The listing builds one solid part. Answer for the finished solid, in the listing's coordinates (mm). Face numbers are marked on the shaded views. Round coordinates to 2 decimals unless told otherwise and drop trailing zeros. Loops run counter-clockwise (first coordinate to the right, second up) from the corner with the lowest first, then second, coordinate; pieces in that order, holes last. Notation, with made-up numbers: (60.25, -27.75) -> (108.25, -27.75) arc R25 cw to (108.25, -2.75) -> close; hole circle Ø7 at (34.25, -13). An arc over 180 degrees is marked (long way). Write each question's results on one line, items separated by ' | '. Start each with the question number.
(1) The part is cut by section D-D (z = -4). Determine the outline of the cut face in (x, y), plus the area to 3 significant figures.
(2) Straight lines are drawn through the part: probe 1 along X at (y, z) = (1.8, 39.5); probe 2 along X at (y, z) = (0.7, 42.5); probe 3 along Y at (x, z) = (-6, -43). For each, find the intervals that lie inside material, in ascending order.
(3) The part is cut by section B-B (x = 23.5). Determine the outline of the cut face in (y, z), plus the area to 3 significant figures.
(4) The part is cut by section C-C (y = 3.3). Determine the outline of the cut face in (x, z), plus the area to 3 significant figures.
(5) Flat-ended cylindrical pins translate along their axes: pin 1 (3 mm diameter, centred on x = 13.5, z = -7.5, fed in from +Y); pin 2 (1.8 mm diameter, centred on x = 13.5, z = 42.5, fed in from -Y). Find the tip coordinate at first contact, or state that the pin passes through.
(6) Determine the mould class of the marked faces 1 and 2 for opening direction X: released by +X, released by -X, zero draft, split by the parting line, or undercut.
(7) The part is cut by section A-A (z = 42.5). Determine the outline of the cut face in (x, y).
```python
from build123d import *

# Parameters (mm, degrees)
ESQUISSE1_W             = 66
ESQUISSE1_H             = 104
BOSS_EXTRU_1_DEPTH      = 1.5875
ESQUISSE2_W             = 104
ESQUISSE2_H             = 4
BOSS_EXTRU_2_DEPTH      = 1.5875
ESQUISSE3_W             = 104
ESQUISSE3_H             = 4
BOSS_EXTRU_3_DEPTH      = 1.5875
CONG_2_R                = 2
CONG_3_R                = 2
ESQUISSE4_R             = 1
ENL_V_MAT_EXTRU_1_DEPTH = 1.5875


with BuildPart() as part:
    # Esquisse1 → Boss.-Extru.1 (new body)
    with BuildSketch(Plane(origin=(0, 0, 0), x_dir=(1, 0, 0), z_dir=(0, 1, 0))):
        Rectangle(ESQUISSE1_W, ESQUISSE1_H)
    extrude(amount=BOSS_EXTRU_1_DEPTH)

    # Esquisse2 → Boss.-Extru.2 (add)
    with BuildSketch(Plane.ZY.offset(33)):
        with Locations((0, 2)):
            Rectangle(ESQUISSE2_W, ESQUISSE2_H)
    extrude(amount=BOSS_EXTRU_2_DEPTH)

    # Esquisse3 → Boss.-Extru.3 (add)
    with BuildSketch(Plane(origin=(33, 0, 0), x_dir=(0, 0, -1), z_dir=(1, 0, 0))):
        with Locations((0, 2)):
            Rectangle(ESQUISSE3_W, ESQUISSE3_H)
    extrude(amount=BOSS_EXTRU_3_DEPTH)

    # Congé2
    cong_2_edges = [part.edges().sort_by_distance(p)[0] for p in [
        (34.5875, 0, 0),
    ]]
    fillet(cong_2_edges, radius=CONG_2_R)

    # Congé3
    cong_3_edges = [part.edges().sort_by_distance(p)[0] for p in [
        (-34.5875, 0, 0),
    ]]
    fillet(cong_3_edges, radius=CONG_3_R)

    # Esquisse4 → Enlèv. mat.-Extru.1 (cut)
    with BuildSketch(Plane(origin=(0, 1.5875, 0), x_dir=(1, 0, 0), z_dir=(0, 1, 0))):
        with Locations(Location((13.5, 7.5, 0), (0, 0, 270))):
            Circle(ESQUISSE4_R)
        with Locations(Location((23.5, 7.5, 0), (0, 0, 270))):
            Circle(ESQUISSE4_R)
        with Locations(Location((23.5, -42.5, 0), (0, 0, 270))):
            Circle(ESQUISSE4_R)
        with Locations(Location((13.5, -42.5, 0), (0, 0, 270))):
            Circle(ESQUISSE4_R)
    extrude(amount=-ENL_V_MAT_EXTRU_1_DEPTH, mode=Mode.SUBTRACT)


solid = part.part
```
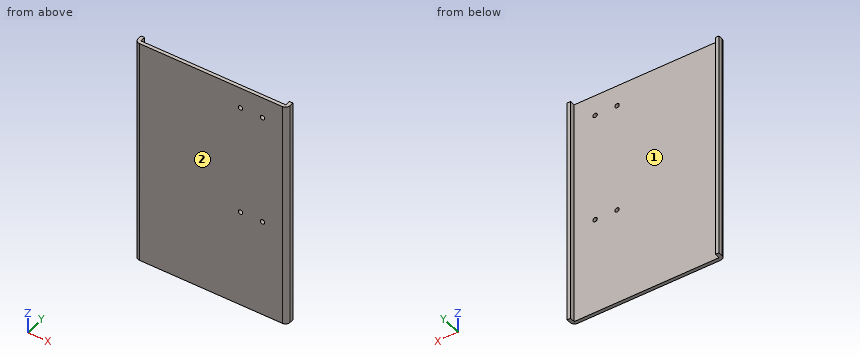
Checked values:
1) outline: (-34.59, 2) arc R2 ccw to (-32.59, 0) -> (32.59, 0) arc R2 ccw to (34.59, 2) -> (34.59, 4) -> (33, 4) -> (33, 1.59) -> (-33, 1.59) -> (-33, 4) -> (-34.59, 4) -> close | area: 116 mm2
2) probe 1: x = -34.58 to -33, 33 to 34.58 | probe 2: x = -34.11 to 12.5, 14.5 to 22.5, 24.5 to 34.11 | probe 3: y = 0 to 1.59
3) outline: (0, -52) -> (1.59, -52) -> (1.59, -8.5) -> (0, -8.5) -> close; (0, -6.5) -> (1.59, -6.5) -> (1.59, 41.5) -> (0, 41.5) -> close; (0, 43.5) -> (1.59, 43.5) -> (1.59, 52) -> (0, 52) -> close | area: 159 mm2
4) outline: (-34.59, -52) -> (-33, -52) -> (-33, 52) -> (-34.59, 52) -> close; (33, -52) -> (34.59, -52) -> (34.59, 52) -> (33, 52) -> close | area: 330 mm2
5) pin 1: stops at y = 1.59 | pin 2: passes through
6) face 1: undercut | face 2: zero draft
7) outline: (-34.59, 2) arc R2 ccw to (-32.59, 0) -> (12.5, 0) -> (12.5, 1.59) -> (-33, 1.59) -> (-33, 4) -> (-34.59, 4) -> close; (14.5, 0) -> (22.5, 0) -> (22.5, 1.59) -> (14.5, 1.59) -> close; (24.5, 0) -> (32.59, 0) arc R2 ccw to (34.59, 2) -> (34.59, 4) -> (33, 4) -> (33, 1.59) -> (24.5, 1.59) -> close
